Check sheet for the modelled part. Datum: model origin and axes. Units: mm. A direction names the side the tool comes from. Coordinates: 2 decimals unless noted, no trailing zeros. Order: outer loops, then holes, each group sorted by start corner. A loop starts at its lowest first (then second) coordinate and runs counter-clockwise, first axis right, second up.
from build123d import *

# Parameters (mm, degrees)
SKETCH1_R           = 60
SKETCH1_R_2         = 1
SKETCH1_W           = 23.5
SKETCH1_H           = 13
BOSS_EXTRUDE1_DEPTH = 3


with BuildPart() as part:
    # Sketch1 → Boss-Extrude1 (new body)
    with BuildSketch(Plane(origin=(0, 0, 0), x_dir=(1, 0, 0), z_dir=(0, 1, 0))):
        with Locations(Location((0, 0, 0), (0, 0, 270))):
            Circle(SKETCH1_R)
        with Locations(Location((26.35, 0, 0), (0, 0, 270))):
            Circle(SKETCH1_R_2, mode=Mode.SUBTRACT)
        with Locations(Location((53.65, 0, 0), (0, 0, 270))):
            Circle(SKETCH1_R_2, mode=Mode.SUBTRACT)
        with Locations(Location((13.175, -22.81976939, 0), (0, 0, 270))):
            Circle(SKETCH1_R_2, mode=Mode.SUBTRACT)
        with Locations(Location((26.825, -46.462262913, 0), (0, 0, 270))):
            Circle(SKETCH1_R_2, mode=Mode.SUBTRACT)
        with Locations(Location((-13.175, -22.81976939, 0), (0, 0, 270))):
            Circle(SKETCH1_R_2, mode=Mode.SUBTRACT)
        with Locations(Location((-26.825, -46.462262913, 0), (0, 0, 270))):
            Circle(SKETCH1_R_2, mode=Mode.SUBTRACT)
        with Locations(Location((-26.35, 0, 0), (0, 0, 270))):
            Circle(SKETCH1_R_2, mode=Mode.SUBTRACT)
        with Locations(Location((-53.65, 0, 0), (0, 0, 270))):
            Circle(SKETCH1_R_2, mode=Mode.SUBTRACT)
        with Locations(Location((-13.175, 22.81976939, 0), (0, 0, 270))):
            Circle(SKETCH1_R_2, mode=Mode.SUBTRACT)
        with Locations(Location((-26.825, 46.462262913, 0), (0, 0, 270))):
            Circle(SKETCH1_R_2, mode=Mode.SUBTRACT)
        with Locations(Location((13.175, 22.81976939, 0), (0, 0, 270))):
            Circle(SKETCH1_R_2, mode=Mode.SUBTRACT)
        with Locations(Location((26.825, 46.462262913, 0), (0, 0, 270))):
            Circle(SKETCH1_R_2, mode=Mode.SUBTRACT)
        with Locations((40, 0)):
            Rectangle(SKETCH1_W, SKETCH1_H, mode=Mode.SUBTRACT)
        Polygon((8.495834875, -27.715217657), (19.754165125, -21.215217657), (31.504165125, -41.566814646), (20.245834875, -48.066814646), align=None, mode=Mode.SUBTRACT)
        Polygon((-19.754165125, -21.215217657), (-8.495834875, -27.715217657), (-20.245834875, -48.066814646), (-31.504165125, -41.566814646), align=None, mode=Mode.SUBTRACT)
        with Locations((-40, 0)):
            Rectangle(SKETCH1_W, SKETCH1_H, mode=Mode.SUBTRACT)
        Polygon((-8.495834875, 27.715217657), (-19.754165125, 21.215217657), (-31.504165125, 41.566814646), (-20.245834875, 48.066814646), align=None, mode=Mode.SUBTRACT)
        Polygon((19.754165125, 21.215217657), (8.495834875, 27.715217657), (20.245834875, 48.066814646), (31.504165125, 41.566814646), align=None, mode=Mode.SUBTRACT)
    extrude(amount=BOSS_EXTRUDE1_DEPTH)


solid = part.part
(1) Tool access check on faces 1 (the flat face through (-51.75, 1, 0)), 2 (the flat face through (1, 3, -1)). Record the directions out of +Z, -Z, +X, -X, +Y, -Y that give a thin tool (end or side, any length) a straight path to the whole face; none if there is none.
Filled in:
face 1: +Y, -Y
face 2: +Z, -Z, +X, -X, +Y
(2) Cross-section at A-A (z = 31). Enter the section's corners in (x, y).
Filled in:
outline: (-51.37, 0) - (-25.4, 0) - (-25.4, 3) - (-51.37, 3) - close; (-10.39, 0) - (10.39, 0) - (10.39, 3) - (-10.39, 3) - close; (25.4, 0) - (51.37, 0) - (51.37, 3) - (25.4, 3) - close
(3) Go/stop test with a flat-tipped pin: P1, Ø1, axis at y = 2, z = 22, coming from the +X side. Record where the tip stops, or that it passes through.
Filled in:
P1: stops at x = 56.02
(4) Release check for a two-part mould opening along X. For faces 3 (the flat face through (-14.05, 1.48, -24.51)), 4 (the cylindrical face through (2.64, 1.48, -59.94)), 5 (the flat face through (1, 0, -1)) record: +X half, -X half, draft (parallel to the pull), parting line (faces both ways), or undercut.
Filled in:
face 3: undercut
face 4: parting line
face 5: draft
(5) Thickness scan on probe 1 along X at (y, z) = (2.65, -30.5); probe 2 along Z at (x, y) = (28, 1.85); probe 3 along Z at (x, y) = (25.5, 2.8). Record the ranges inside material, lowest first.
Filled in:
probe 1: x = -51.67 to -25.11, -10.1 to 10.1, 25.11 to 51.67
probe 2: z = -53.07 to -43.59, -35.5 to 35.5, 43.59 to 53.07
probe 3: z = -54.31 to -45.03, -31.17 to -0.53, 0.53 to 31.17, 45.03 to 54.31
(6) Cross-section at D-D (y = 1.95). Count the separate pieces of the cut face and the enclosed holes in it, and give its area (3 significant figures).
Filled in:
separate pieces: 1
enclosed holes: 18
area: 9,440 mm2
(7) Cross-section at C-C (z = 43). Enter the section's corners in (x, y), and give its area (3 significant figures).
Filled in:
outline: (-41.84, 0) - (-29.02, 0) - (-29.02, 3) - (-41.84, 3) - close; (-17.32, 0) - (17.32, 0) - (17.32, 3) - (-17.32, 3) - close; (29.02, 0) - (41.84, 0) - (41.84, 3) - (29.02, 3) - close
area: 181 mm2
(8) Cross-section at B-B (x = -40). Enter the section's corners in (y, z).
Filled in:
outline: (0, -44.72) - (3, -44.72) - (3, -6.5) - (0, -6.5) - close; (0, 6.5) - (3, 6.5) - (3, 44.72) - (0, 44.72) - close
